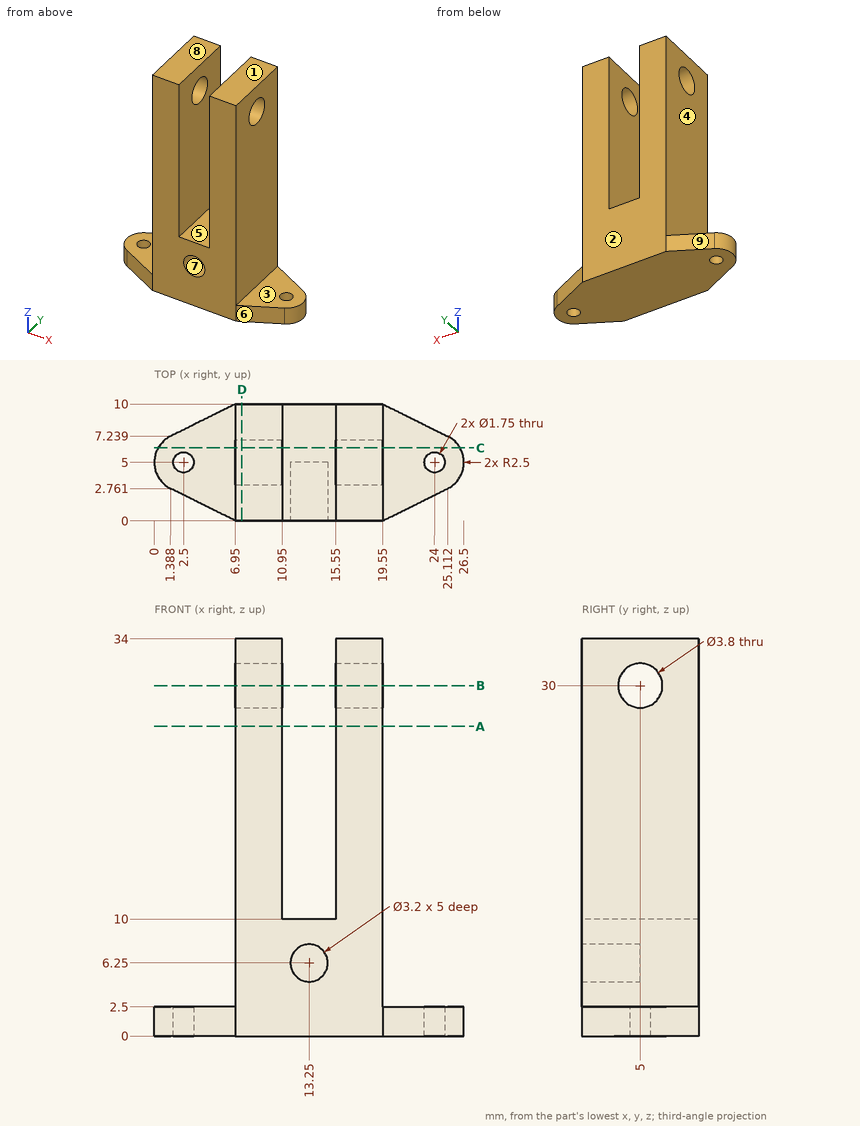
The figure shows three views and two pictorial views of one solid part (mm, origin at its lowest corner). Answer the questions. A direction names the side the tool comes from. Give positions to 0.01 mm unless a question says otherwise; leave off trailing zeros. Loops run counter-clockwise (first coordinate to the right, second up) from the corner with the lowest first, then second, coordinate; pieces in that order, holes last. Notation, with made-up numbers: (7.25, -17) -> (37.25, -17) arc R12 cw to (37.25, 5) -> close; hole circle Ø11 at (66.5, 34.5). An arc over 180 degrees is marked (long way). Use a Markdown table: item, result. Add a question column.
1. Section B-B on z = 30 is taken. Determine the outline of the cut face in (x, y), and give its area (3 significant figures).
2. Flat-ended cylindrical pins translate along their axes: pin 1 Ø1 at (y, z) = (5.5, 15.5) entering from -X; pin 2 Ø6 at (x, y) = (11.5, 6) entering from +Z; pin 3 Ø3 at (x, z) = (13.25, 6.25) entering from -Y; pin 4 Ø1.5 at (y, z) = (4, 27.5) entering from +X. Find the tip coordinate at first contact, or state that the pin passes through.
3. Section A-A on z = 26.5 is taken. Determine the outline of the cut face in (x, y).
4. Determine the mould class of the marked faces 6, 7, 8 and 9 for opening direction X: released by +X, released by -X, zero draft, split by the parting line, or undercut.
5. For the marked faces 1, 2, 3, 4 and 5, determine the directions among +Z, -Z, +X, -X, +Y, -Y from which every point of the face is accessible in a straight line to the end or side of a thin tool.
6. Find the intervals of material crossed by probe 1 along X at (y, z) = (5, 1) (1 decimal); probe 2 along X at (y, z) = (1.75, 25); probe 3 along Z at (x, y) = (16.4, 5), in increasing order.
7. Section D-D on x = 7.5 is taken. Determine the outline of the cut face in (y, z), and give its area (3 significant figures).
8. Section C-C on y = 6.25 is taken. State how many separate pieces and enclosed holes the cut face has, and give its area (3 significant figures).
Results below:
| question | item | result |
|---|---|---|
| 1 | outline | (6.95, 0) -> (10.95, 0) -> (10.95, 3.1) -> (6.95, 3.1) -> close; (6.95, 6.9) -> (10.95, 6.9) -> (10.95, 10) -> (6.95, 10) -> close; (15.55, 0) -> (19.55, 0) -> (19.55, 3.1) -> (15.55, 3.1) -> close; (15.55, 6.9) -> (19.55, 6.9) -> (19.55, 10) -> (15.55, 10) -> close |
| 1 | area | 49.6 mm^2 |
| 2 | pin 1 | stops at x = 6.95 |
| 2 | pin 2 | stops at z = 34 |
| 2 | pin 3 | stops at y = 5 |
| 2 | pin 4 | stops at x = 19.55 |
| 3 | outline | (6.95, 0) -> (10.95, 0) -> (10.95, 10) -> (6.95, 10) -> close; (15.55, 0) -> (19.55, 0) -> (19.55, 10) -> (15.55, 10) -> close |
| 4 | face 6 | released by +X |
| 4 | face 7 | undercut |
| 4 | face 8 | zero draft |
| 4 | face 9 | released by -X |
| 5 | face 1 | +Z, +X, -X, +Y, -Y |
| 5 | face 2 | +Z, -Z, +X, -X, +Y |
| 5 | face 3 | +Z, +X, +Y, -Y |
| 5 | face 4 | +Z, -X, +Y, -Y |
| 5 | face 5 | +Z, +Y, -Y |
| 6 | probe 1 | x = 0 to 1.6, 3.4 to 23.1, 24.9 to 26.5 |
| 6 | probe 2 | x = 6.95 to 10.95, 15.55 to 19.55 |
| 6 | probe 3 | z = 0 to 28.1, 31.9 to 34 |
| 7 | outline | (0, 0) -> (10, 0) -> (10, 34) -> (0, 34) -> close; hole circle Ø3.8 at (5, 30) |
| 7 | area | 329 mm^2 |
| 8 | separate pieces | 3 |
| 8 | enclosed holes | 0 |
| 8 | area | 328 mm^2 |
